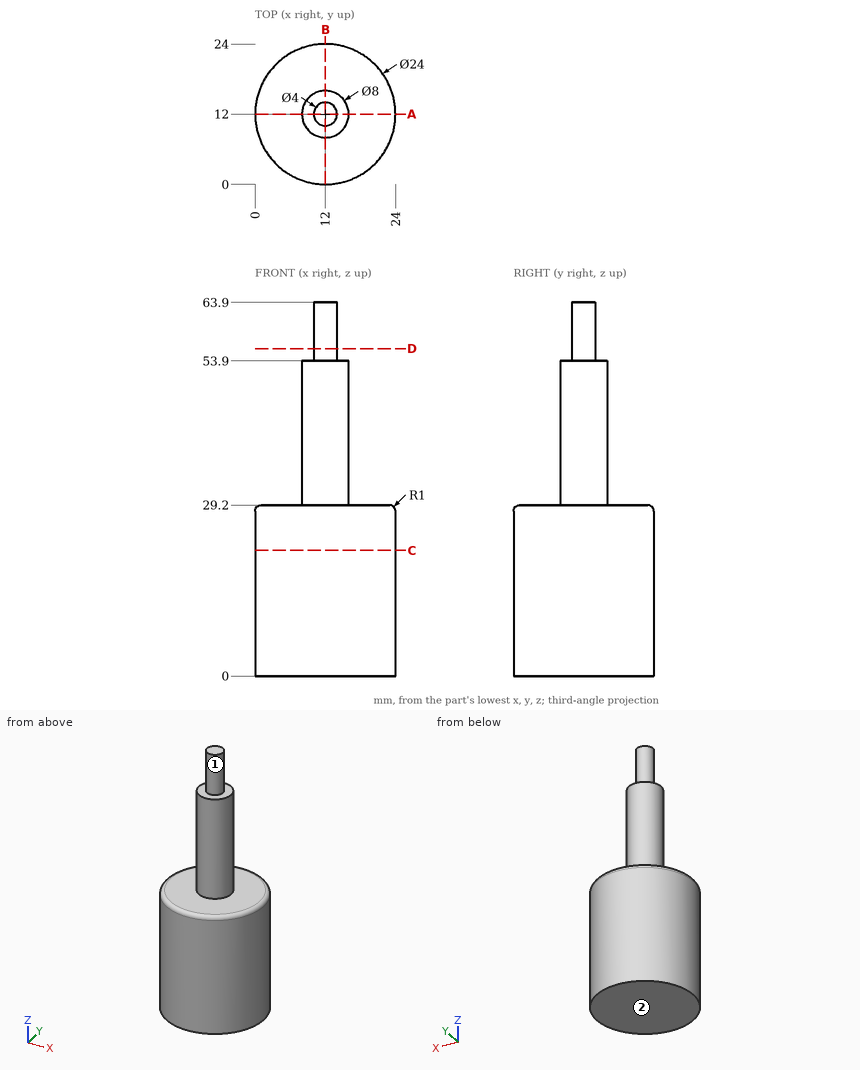
Verification items for this drawing (mm, ordinates from the low corner). A direction names the side the tool comes from. Give positions to 0.01 mm unless a question says otherwise; leave off trailing zeros. Loops run counter-clockwise (first coordinate to the right, second up) from the corner with the lowest first, then second, coordinate; pieces in that order, holes last. Notation, with made-up numbers: M 25,-36 L 68,-36 A18 cw 68,-28 Z; hole C 19.5,30 d8. An arc over 180 degrees is marked long. Answer as a JSON object with one key per item and string values. Group by question number.
Q1. Cross-section at D-D on z = 56. Record the cut outline in (x, y), then the cut area to 3 significant figures.
Q2. Go/stop test with flat-tipped pins: P1, Ø5, axis at y = 10.5, z = 53, coming from the -X side; P2, Ø2, axis at x = 7, z = 12.5, coming from the -Y side. Record where each tip stops, or that it passes through.
Q3. Cross-section at C-C on z = 21.5. Record the cut outline in (x, y), then the cut area to 3 significant figures.
Q4. Material ranges on line 1 along Z through (x, y) = (22.25, 12); line 2 along Z through (x, y) = (13.5, 9.75); line 3 along X through (y, z) = (13.5, 13.5), recorded low to high. Write a range as [from, to].
Q5. Access from +Z, -Z, +X, -X, +Y, -Y to the whole of each face (thin tool, end or side, straight path). Record for the marked faces 1 and 2.
Q6. Cross-section at A-A on y = 12. Record the cut outline in (x, z).
Evaluation:
{
 "1": {"outline": "C 12,12 d4", "area": "12.6 mm2"},
 "2": {"P1": "stops at x = 8", "P2": "stops at y = 0.69"},
 "3": {"outline": "C 12,12 d24", "area": "452 mm2"},
 "4": {"line 1": "z = [0, 29.2]", "line 2": "z = [0, 53.9]", "line 3": "x = [0.09, 23.91]"},
 "5": {"face 1": "+Z", "face 2": "-Z, +X, -X, +Y, -Y"},
 "6": {"outline": "M 0,0 L 24,0 L 24,28.2 A1 ccw 23,29.2 L 16,29.2 L 16,53.9 L 14,53.9 L 14,63.9 L 10,63.9 L 10,53.9 L 8,53.9 L 8,29.2 L 1,29.2 A1 ccw 0,28.2 Z"}
}
